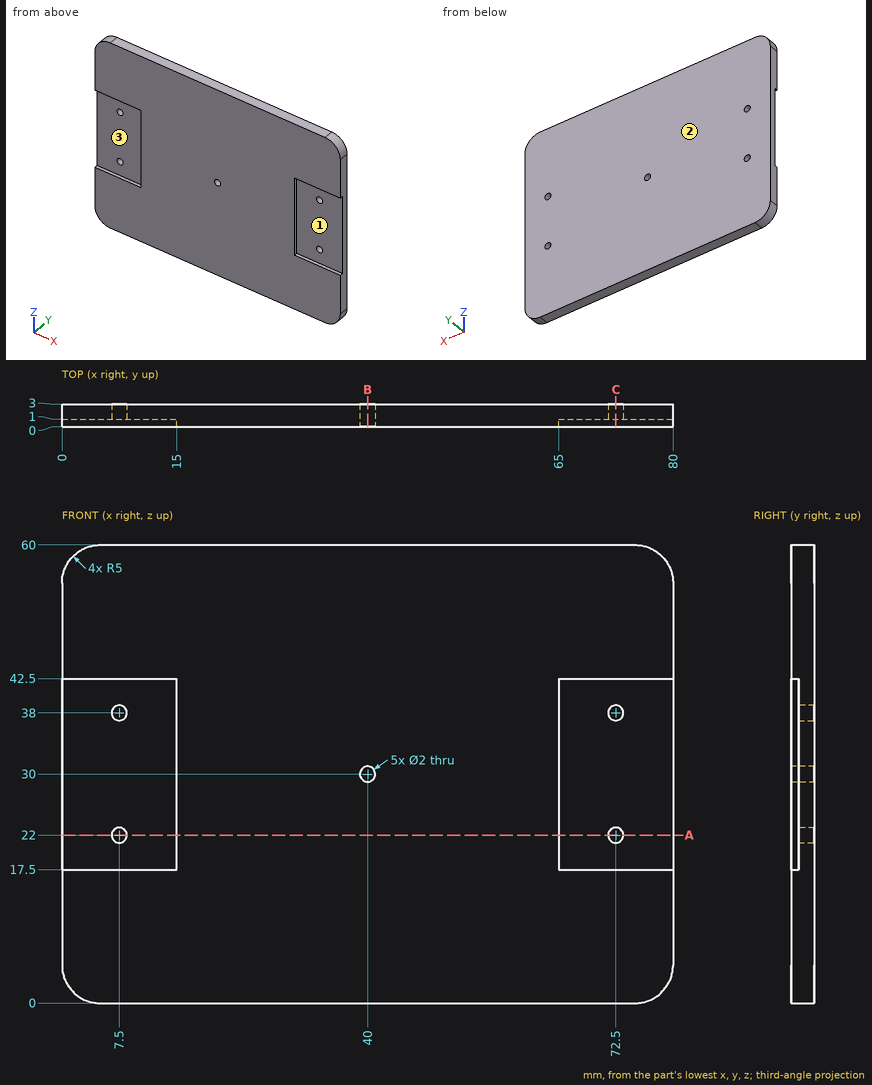
Drawing for the job (mm, zero at the part's lowest x, y, z). Round coordinates to 2 decimals unless told otherwise and drop trailing zeros. Loops run counter-clockwise (first coordinate to the right, second up) from the corner with the lowest first, then second, coordinate; pieces in that order, holes last. Notation, with made-up numbers: (18.25, 33.25) -> (74.25, 33.25) arc R10 ccw to (74.25, 46.25) -> close; hole circle Ø5 at (63, 21.5). An arc over 180 degrees is marked (long way). Answer as CSV lines item,"result". Start each with the question number.
1) Probe line 1 along Z through (x, y) = (72.5, 2.35); line 2 along X through (y, z) = (2.2, 22); line 3 along X through (y, z) = (0.4, 30). List the from-to ranges inside material, lowest first.
2) Pin check, flat tip, straight feed: P1, Ø7.5, axis at x = 7, z = 24, coming from the -Y side. Stop position of the tip, or through.
3) Slice it at A-A (z = 22). List the corners of the cut face in (x, y), plus the area to 3 significant figures.
4) Slice it at C-C (x = 72.5). List the corners of the cut face in (y, z), plus the area to 3 significant figures.
5) Slice it at B-B (x = 40). List the corners of the cut face in (y, z), plus the area to 3 significant figures.
6) Mould opens along Z. For the marked faces 1, 2 and 3 say: +Z half, -Z half, draft (parallel to the pull), parting line (faces both ways), or undercut.
Filled in:
1,line 1,"z = 0 to 21, 23 to 37, 39 to 60"
1,line 2,"x = 0 to 6.5, 8.5 to 71.5, 73.5 to 80"
1,line 3,"x = 15 to 39, 41 to 65"
2,P1,"stops at y = 1"
3,outline,"(0, 1) -> (6.5, 1) -> (6.5, 3) -> (0, 3) -> close; (8.5, 1) -> (15, 1) -> (15, 0) -> (65, 0) -> (65, 1) -> (71.5, 1) -> (71.5, 3) -> (8.5, 3) -> close; (73.5, 1) -> (80, 1) -> (80, 3) -> (73.5, 3) -> close"
3,area,"202 mm2"
4,outline,"(0, 0) -> (3, 0) -> (3, 21) -> (1, 21) -> (1, 17.5) -> (0, 17.5) -> close; (0, 42.5) -> (1, 42.5) -> (1, 39) -> (3, 39) -> (3, 60) -> (0, 60) -> close; (1, 23) -> (3, 23) -> (3, 37) -> (1, 37) -> close"
4,area,"147 mm2"
5,outline,"(0, 0) -> (3, 0) -> (3, 29) -> (0, 29) -> close; (0, 31) -> (3, 31) -> (3, 60) -> (0, 60) -> close"
5,area,"174 mm2"
6,face 1,"undercut"
6,face 2,"draft"
6,face 3,"undercut"
